Could you check a few things on this model? Use its own coordinates, in mm. Round coordinates to 2 decimals unless told otherwise and drop trailing zeros. Order: outer loops, then holes, each group sorted by start corner. A loop starts at its lowest first (then second) coordinate and runs counter-clockwise, first axis right, second up. Notation, with made-up numbers: (15.5, 71.25) - (46.5, 71.25) arc R18 cw to (46.5, 78.25) - close; hole circle Ø2 at (38, -4). An arc over 180 degrees is marked (long way). Return JSON: item names as keys, results as strings. Group by question number.
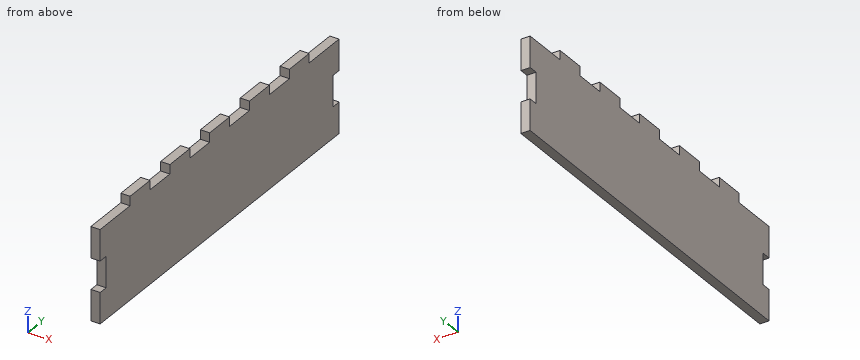
from build123d import *

# Parameters (mm, degrees)
F0_W     = 6
F0_H     = 240
F1_DEPTH = 60
F2_W     = 6
F2_H     = 20
F3_DEPTH = 6.001
F2_W_2   = 20
F2_H_2   = 6
F4_DEPTH = 6


with BuildPart() as f1:
    # F0 (on Top) → F1 (new body)
    with BuildSketch(Plane.XY):
        Rectangle(F0_W, F0_H)
    extrude(amount=F1_DEPTH)

    # F2 (on face) → F3 (cut, through all)
    with BuildSketch(Plane(origin=(-3, 0, 0), x_dir=(0, -1, 0), z_dir=(-1, 0, 0))):
        with Locations((-117, 30)):
            Rectangle(F2_W, F2_H)
        with Locations((117, 30)):
            Rectangle(F2_W, F2_H)
    extrude(amount=-F3_DEPTH, mode=Mode.SUBTRACT)

    # F2 (on face) → F4 (join)
    with BuildSketch(Plane(origin=(-3, 0, 0), x_dir=(0, -1, 0), z_dir=(-1, 0, 0))):
        with Locations((80, 63)):
            Rectangle(F2_W_2, F2_H_2)
        with Locations((40, 63)):
            Rectangle(F2_W_2, F2_H_2)
        with Locations((0, 63)):
            Rectangle(F2_W_2, F2_H_2)
        with Locations((-40, 63)):
            Rectangle(F2_W_2, F2_H_2)
        with Locations((-80, 63)):
            Rectangle(F2_W_2, F2_H_2)
    extrude(amount=-F4_DEPTH)


solid = f1.part
1) I want a section at C-C, the plane y = -103. List the corners of the cut face in (x, z) for me.
2) If I drill on line 1 along Y through (x, z) = (-0.15, 60.5); line 2 along Y through (x, z) = (0, 31.5); line 3 along Z through (x, y) = (-2.1, 66.5), over which ranges is the centre line in solid material (lowest first)? Write a range as from..to.
3) Will these pins go through, and if not, where does the flat tip stop? pin 1 (3 mm diameter, centred on x = 0.5, y = 111, fed in from +Z); pin 2 (1.8 mm diameter, centred on x = 0.5, z = 30.5, fed in from +Y); pin 3 (3 mm diameter, centred on x = 1, z = 64, fed in from -Y).
4) I want a section at B-B, the plane z = 25.5. List the corners of the cut face in (x, y) for me, plus the area to 3 significant figures.
Outcome:
{
 "1": {"outline": "(-3, 0) - (3, 0) - (3, 60) - (-3, 60) - close"},
 "2": {"line 1": "-90..-70, -50..-30, -10..10, 30..50, 70..90", "line 2": "-114..114", "line 3": "0..60"},
 "3": {"pin 1": "z = 60", "pin 2": "y = 114", "pin 3": "y = -90"},
 "4": {"outline": "(-3, -114) - (3, -114) - (3, 114) - (-3, 114) - close", "area": "1,370 mm^2"}
}
